The drawing under review shows one solid part. Ordinate dimensions are in mm from its lowest x, y, z. Coordinates: 2 decimals unless noted, no trailing zeros. Order: outer loops, then holes, each group sorted by start corner. A loop starts at its lowest first (then second) coordinate and runs counter-clockwise, first axis right, second up. Notation, with made-up numbers: (9, -12.75) -> (41, -12.75) arc R20 cw to (41, 8.25) -> close; hole circle Ø11 at (-11.5, 86.5). An arc over 180 degrees is marked (long way). Use a Markdown table: item, result. Add a question column.
Q1. Add section D-D (y = 4). State the section outline as (x, z) points.
Q2. Wall thickness on probe 1 along X at (y, z) = (18, 0.25); probe 2 along X at (y, z) = (18.5, 2.05); probe 3 along X at (y, z) = (8.5, 1.2): over which ranges is each line inside the solid? List them lowest first.
Q3. Add section A-A (y = 21). State the section outline as (x, z) points, then the cut area to 3 significant figures.
Q4. Add section B-B (z = 1.3). State the section outline as (x, y) points.
Q5. The part is to be moulded in two halves that separate along X. For the marked faces 1 and 2, say which applies: pulls with the +X half, pulls with the -X half, needs draft (parallel to the pull), parting line crosses it, or undercut.
Q6. Insertion check: pin 1 (6 mm diameter, centred on x = 27, y = 28, fed in from -Z); pin 2 (0.8 mm diameter, centred on x = 44, z = 2, fed in from -Y); pin 3 (0.8 mm diameter, centred on y = 11.5, z = 1, fed in from -X). Each pin has a flat end and moves straight along its axis. Give the tip position at first contact, or say it passes through.
Q7. Add section C-C (x = 38.1). State the section outline as (y, z) points, then the cut area to 3 significant figures.
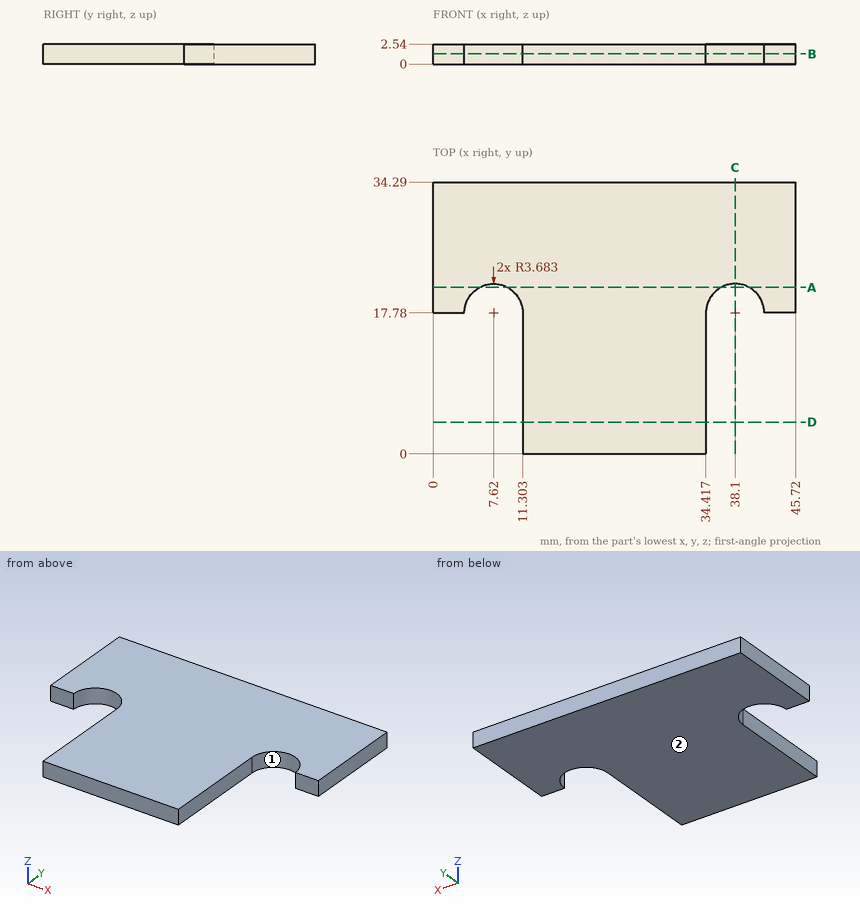
Established:
| question | item | result |
|---|---|---|
| 1 | outline | (11.3, 0) -> (34.42, 0) -> (34.42, 2.54) -> (11.3, 2.54) -> close |
| 2 | probe 1 | 0 to 3.94, 11.3 to 34.42, 41.78 to 45.72 |
| 2 | probe 2 | 0 to 4.01, 11.23 to 34.49, 41.71 to 45.72 |
| 2 | probe 3 | 11.3 to 34.42 |
| 3 | outline | (0, 0) -> (5.83, 0) -> (5.83, 2.54) -> (0, 2.54) -> close; (9.41, 0) -> (36.31, 0) -> (36.31, 2.54) -> (9.41, 2.54) -> close; (39.89, 0) -> (45.72, 0) -> (45.72, 2.54) -> (39.89, 2.54) -> close |
| 3 | area | 98.0 mm^2 |
| 4 | outline | (0, 17.78) -> (3.94, 17.78) arc R3.68 cw to (11.3, 17.78) -> (11.3, 0) -> (34.42, 0) -> (34.42, 17.78) arc R3.68 cw to (41.78, 17.78) -> (45.72, 17.78) -> (45.72, 34.29) -> (0, 34.29) -> close |
| 5 | face 1 | undercut |
| 5 | face 2 | needs draft |
| 6 | pin 1 | z = 0 |
| 6 | pin 2 | y = 17.78 |
| 6 | pin 3 | x = 11.3 |
| 7 | outline | (21.46, 0) -> (34.29, 0) -> (34.29, 2.54) -> (21.46, 2.54) -> close |
| 7 | area | 32.6 mm^2 |
